Design review of the part shown in the three views and the two pictorial views. Dimensions are in mm from the part's minimum x, y and z. Coordinates: 2 decimals unless noted, no trailing zeros. Order: outer loops, then holes, each group sorted by start corner. A loop starts at its lowest first (then second) coordinate and runs counter-clockwise, first axis right, second up. Notation, with made-up numbers: (48.25, 41.25) -> (65.25, 41.25) arc R31 cw to (65.25, 71.25) -> close; hole circle Ø11 at (85.25, -29.5). An arc over 180 degrees is marked (long way). Answer as a JSON object with one key per item and string values. Group by question number.
1) Draft analysis for pull direction Y (two halves, no side actions). For the marked faces 1 and 2, state which applies: +Y half, -Y half, draft (parallel to the pull), parting line (faces both ways), or undercut.
2) Wall thickness on L1, parallel to X at y = 103, z = 28.5; L2, parallel to X at y = 29, z = 29.5; L3, parallel to Z at x = 79, y = 81.5: over which ranges is each line inside the solid? List them lowest first.
3) Add section A-A, the plane z = 26. Write out the cut boundary in (x, y), then the cut area to 3 significant figures.
4) Add section C-C, the plane x = 183.5. Write out the cut boundary in (y, z), then the cut area to 3 significant figures.
5) For pin 1 (9.5 mm diameter, centred on x = 243, z = 27.5, fed in from -Y); pin 2 (2 mm diameter, centred on x = 222, y = 74.5, fed in from -Z); pin 3 (5.5 mm diameter, centred on y = 79, z = 24, fed in from -X); pin 4 (5 mm diameter, centred on x = 157, z = 32, fed in from +Y), all flat-tipped, find the tip position at first contact; note any pin that passes through.
6) Add section D-D, the plane y = 21. Write out the cut boundary in (x, z), then the cut area to 3 significant figures.
7) Add section B-B, the plane y = 94. Write out the cut boundary in (x, z).
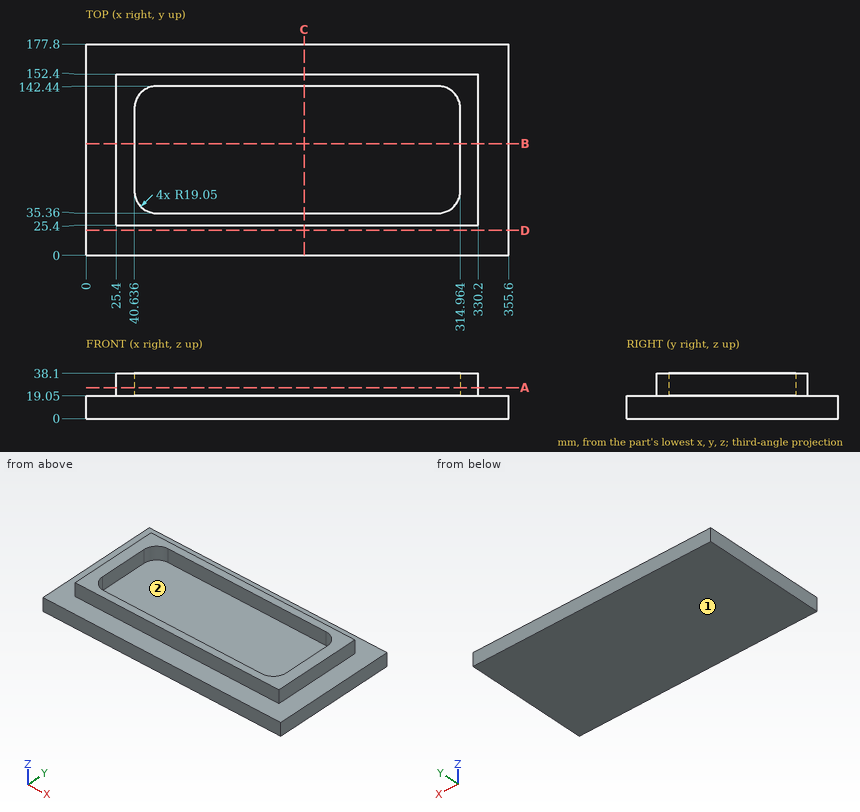
Output values:
{
 "1": {"face 1": "draft", "face 2": "undercut"},
 "2": {"L1": "x = 25.4 to 40.64, 314.96 to 330.2", "L2": "x = 25.4 to 330.2", "L3": "z = 0 to 19.05"},
 "3": {"outline": "(25.4, 25.4) -> (330.2, 25.4) -> (330.2, 152.4) -> (25.4, 152.4) -> close; hole (40.64, 54.41) arc R19.05 ccw to (59.69, 35.36) -> (295.91, 35.36) arc R19.05 ccw to (314.96, 54.41) -> (314.96, 123.39) arc R19.05 ccw to (295.91, 142.44) -> (59.69, 142.44) arc R19.05 ccw to (40.64, 123.39) -> close", "area": "9,650 mm²"},
 "4": {"outline": "(0, 0) -> (177.8, 0) -> (177.8, 19.05) -> (152.4, 19.05) -> (152.4, 38.1) -> (142.44, 38.1) -> (142.44, 19.05) -> (35.36, 19.05) -> (35.36, 38.1) -> (25.4, 38.1) -> (25.4, 19.05) -> (0, 19.05) -> close", "area": "3,770 mm²"},
 "5": {"pin 1": "stops at y = 25.4", "pin 2": "stops at z = 0", "pin 3": "stops at x = 25.4", "pin 4": "stops at y = 152.4"},
 "6": {"outline": "(0, 0) -> (355.6, 0) -> (355.6, 19.05) -> (0, 19.05) -> close", "area": "6,770 mm²"},
 "7": {"outline": "(0, 0) -> (355.6, 0) -> (355.6, 19.05) -> (330.2, 19.05) -> (330.2, 38.1) -> (314.96, 38.1) -> (314.96, 19.05) -> (40.64, 19.05) -> (40.64, 38.1) -> (25.4, 38.1) -> (25.4, 19.05) -> (0, 19.05) -> close"}
}
